Geometry: final body of the model. Coordinates: model frame, mm. A direction names the side the tool comes from. Coordinates: 2 decimals unless noted, no trailing zeros. Write each loop counter-clockwise with the first axis right and the second up, starting at its lowest first coordinate (ties: lowest second). Pieces come first, ordered by that corner, then holes. Notation, with made-up numbers: (20, -9) -> (62, -9) arc R27 cw to (62, 7) -> close; hole circle Ø11 at (57, 6.25). An arc over 180 degrees is marked (long way). One line per item, written item: value.
```python
from build123d import *

# Parameters (mm, degrees)
SKETCH1_R               = 2
SKETCH1_R_2             = 8.2
BOSS_EXTRUDE1_DEPTH     = 2
SKETCH3_W               = 59.6
SKETCH3_H               = 25
SKETCH3_R               = 2
SKETCH3_W_2             = 46
SKETCH3_H_2             = 21
BOSS_EXTRUDE3_DEPTH     = 7
CUT_EXTRUDE1_DEPTH      = 40.925430492
CUT_EXTRUDE1_DEPTH_BACK = 3


with BuildPart() as part:
    # Sketch1 → Boss-Extrude1 (new body)
    with BuildSketch(Plane(origin=(0, 0, 0), x_dir=(0, 0, -1), z_dir=(1, 0, 0))):
        Polygon((25, 12.5), (-25, 12.5), (-29.8, 12.5), (-29.8, -12.5), (-25, -12.5), (25, -12.5), (29.8, -12.5), (29.8, 12.5), align=None)
        with Locations((-26.5, 0)):
            Circle(SKETCH1_R, mode=Mode.SUBTRACT)
        with Locations((-13.2, 0)):
            Circle(SKETCH1_R_2, mode=Mode.SUBTRACT)
        with Locations((13.2, 0)):
            Circle(SKETCH1_R_2, mode=Mode.SUBTRACT)
        with Locations((26.5, 0)):
            Circle(SKETCH1_R, mode=Mode.SUBTRACT)
    extrude(amount=BOSS_EXTRUDE1_DEPTH)

    # Sketch3 → Boss-Extrude3 (add)
    with BuildSketch(Plane(origin=(2, 0, 0), x_dir=(0, 0, -1), z_dir=(1, 0, 0))):
        Rectangle(SKETCH3_W, SKETCH3_H)
        with Locations((-26.5, 0)):
            Circle(SKETCH3_R, mode=Mode.SUBTRACT)
        with Locations((26.5, 0)):
            Circle(SKETCH3_R, mode=Mode.SUBTRACT)
        Rectangle(SKETCH3_W_2, SKETCH3_H_2, mode=Mode.SUBTRACT)
    extrude(amount=BOSS_EXTRUDE3_DEPTH)

    # Sketch5 → Cut-Extrude1 (cut, two sides: drawn at the far end of the back side and taken through both)
    with BuildSketch(Plane(origin=(0, 12.5, 0), x_dir=(1, 0, 0), z_dir=(0, 1, 0)).offset(-CUT_EXTRUDE1_DEPTH_BACK)):
        Polygon((92.827908002, 6), (9, 6), (6, 6), (6, -6), (9, -6), (92.827908002, -6), (260.483724007, -6), (260.483724007, 6), align=None)
    extrude(amount=CUT_EXTRUDE1_DEPTH + CUT_EXTRUDE1_DEPTH_BACK, mode=Mode.SUBTRACT)


solid = part.part
```
(1) Section C-C (y = 0). Return the cut outline in (x, z), then the cut area to 3 significant figures.
Responses:
outline: (0, -29.8) -> (9, -29.8) -> (9, -28.5) -> (0, -28.5) -> close; (0, -24.5) -> (9, -24.5) -> (9, -23) -> (2, -23) -> (2, -21.4) -> (0, -21.4) -> close; (0, -5) -> (2, -5) -> (2, 5) -> (0, 5) -> close; (0, 21.4) -> (2, 21.4) -> (2, 23) -> (9, 23) -> (9, 24.5) -> (0, 24.5) -> close; (0, 28.5) -> (9, 28.5) -> (9, 29.8) -> (0, 29.8) -> close
area: 76.8 mm2
(2) Section D-D (y = 4.25). Return the cut outline in (x, z).
Responses:
outline: (0, -29.8) -> (9, -29.8) -> (9, -23) -> (2, -23) -> (2, -20.21) -> (0, -20.21) -> close; (0, -6.19) -> (2, -6.19) -> (2, 6.19) -> (0, 6.19) -> close; (0, 20.21) -> (2, 20.21) -> (2, 23) -> (9, 23) -> (9, 29.8) -> (0, 29.8) -> close
(3) Reachability of faces 4 (the flat face through (8, 11, -6)), 5 (the flat face through (5, 0, -23)), 6 (the flat face through (0, 0, 0)) from +Z, -Z, +X, -X, +Y, -Y: full face, straight path, thin tool, end or side. Return the list, or none.
Responses:
face 4: +X, +Y
face 5: +X
face 6: +Z, -Z, -X, +Y, -Y
(4) Pull-direction query (Z, two-part tool) for faces 1 (the flat face through (4, 12.5, 0)), 2 (the flat face through (7, 11, 6)), 3 (the flat face through (4, 0, 29.8)); classes: released by +Z, released by -Z, zero draft, split by the parting line, or undercut.
Responses:
face 1: zero draft
face 2: undercut
face 3: released by +Z
(5) Section A-A (z = 26.5). Return the cut outline in (x, y), then the cut area to 3 significant figures.
Responses:
outline: (0, -12.5) -> (9, -12.5) -> (9, -2) -> (0, -2) -> close; (0, 2) -> (9, 2) -> (9, 12.5) -> (0, 12.5) -> close
area: 189 mm2
(6) Section B-B (x = 1). Return the cut outline in (y, z).
Responses:
outline: (-12.5, -29.8) -> (12.5, -29.8) -> (12.5, 29.8) -> (-12.5, 29.8) -> close; hole circle Ø16.4 at (0, -13.2); hole circle Ø16.4 at (0, 13.2); hole circle Ø4 at (0, -26.5); hole circle Ø4 at (0, 26.5)
(7) Line query: line 1 (Y direction, x = 4.5, z = 14.5); line 2 (Y direction, x = 1.25, z = -13.2); line 3 (Z direction, x = 3.75, y = 9). Output: solid intervals per line, ascending. Write a range as [from, to].
Responses:
line 1: y = [-12.5, -10.5], [10.5, 12.5]
line 2: y = [-12.5, -8.2], [8.2, 12.5]
line 3: z = [-29.8, -23], [23, 29.8]
(8) First-contact query: pin 1 (2.5 mm diameter, centred on y = 0, z = 26.5, fed in from -X); pin 2 (2 mm diameter, centred on y = 11, z = 0.5, fed in from +X). Flat tips, straight axial feed; report the tip coordinate or a pass-through.
Responses:
pin 1: passes through
pin 2: stops at x = 6
